Geometry: final body of the model. Coordinates: model frame, mm. A direction names the side the tool comes from. Coordinates: 2 decimals unless noted, no trailing zeros. Loops run counter-clockwise (first coordinate to the right, second up) from the corner with the lowest first, then second, coordinate; pieces in that order, holes last. Notation, with made-up numbers: (1, 54) - (52, 54) arc R33 cw to (52, 83) - close; hole circle Ø9 at (52, 58). An arc over 180 degrees is marked (long way). Answer in a Markdown table with one row per item.
from build123d import *

# Parameters (mm, degrees)
SKETCH1_W           = 100
SKETCH1_H           = 200
BOSS_EXTRUDE1_DEPTH = 5
SKETCH2_R           = 4.9
BOSS_EXTRUDE2_DEPTH = 10


with BuildPart() as part:
    # Sketch1 → Boss-Extrude1 (new body)
    with BuildSketch(Plane.XY):
        with Locations((50, 100)):
            Rectangle(SKETCH1_W, SKETCH1_H)
    extrude(amount=BOSS_EXTRUDE1_DEPTH)

    # Sketch2 → Boss-Extrude2 (add)
    with BuildSketch(Plane.XY.offset(5)):
        with Locations(Location((17.5, 10, 0), (0, 0, 180))):
            Circle(SKETCH2_R)
        with Locations(Location((77.5, 190, 0), (0, 0, 180))):
            Circle(SKETCH2_R)
    extrude(amount=BOSS_EXTRUDE2_DEPTH)


solid = part.part
(1) Pull-direction query (X, two-part tool) for faces 1 (the face through (100, 99, 2)), 2 (the face through (49, 200, 2)), 3 (the face through (0, 99, 2)); classes: pulls with the +X half, pulls with the -X half, needs draft (parallel to the pull), parting line crosses it, or undercut.
Verdict:
| item | result |
|---|---|
| face 1 | pulls with the +X half |
| face 2 | needs draft |
| face 3 | pulls with the -X half |
(2) Access query for faces 4 (the face through (49, 0, 2)), 5 (the face through (18.14, 5.14, 9.93)). Directions: +Z, -Z, +X, -X, +Y, -Y. A direction counts if a zero-diameter tool reaches every point of the face in a straight line with its end or side. Return the directions, or none.
Verdict:
| item | result |
|---|---|
| face 4 | +Z, -Z, +X, -X, -Y |
| face 5 | +Z |
(3) Cut plane B-B on y = 10. Output: boundary loops of the cut face in (x, z), then the cut area to 3 significant figures.
Verdict:
| item | result |
|---|---|
| outline | (0, 0) - (100, 0) - (100, 5) - (22.4, 5) - (22.4, 15) - (12.6, 15) - (12.6, 5) - (0, 5) - close |
| area | 598 mm² |
(4) Ray query, probe 1 along Z at (x, y) = (68, 113.5); probe 2 along X at (y, z) = (190, 5.75); probe 3 along Y at (x, z) = (73, 9.5). Return the intervals inside material, ascending.
Verdict:
| item | result |
|---|---|
| probe 1 | z = 0 to 5 |
| probe 2 | x = 72.6 to 82.4 |
| probe 3 | y = 188.06 to 191.94 |
(5) Cut plane A-A on x = 77.5. Output: boundary loops of the cut face in (y, z).
Verdict:
| item | result |
|---|---|
| outline | (0, 0) - (200, 0) - (200, 5) - (194.9, 5) - (194.9, 15) - (185.1, 15) - (185.1, 5) - (0, 5) - close |
(6) First-contact query: pin 1 Ø10 at (x, y) = (10.5, 49) entering from +Z; pin 2 Ø1 at (x, z) = (78.5, 6) entering from -Y. Flat tips, straight axial feed; report the tip coordinate or a pass-through.
Verdict:
| item | result |
|---|---|
| pin 1 | stops at z = 5 |
| pin 2 | stops at y = 185.13 |
(7) Cut plane C-C on z = 7. Output: boundary loops of the cut face in (x, y).
Verdict:
| item | result |
|---|---|
| outline | circle Ø9.8 at (17.5, 10); circle Ø9.8 at (77.5, 190) |
(8) Cut plane D-D on x = 28. Output: boundary loops of the cut face in (y, z), then the cut area to 3 significant figures.
Verdict:
| item | result |
|---|---|
| outline | (0, 0) - (200, 0) - (200, 5) - (0, 5) - close |
| area | 1,000 mm² |
